Autodesk Inventor part; units mm, degrees
ref_plane "YZ Plane" through (0, 0, 0) normal (1, 0, 0) x (0, 1, 0)
ref_plane "XZ Plane" through (0, 0, 0) normal (0, 1, 0) x (-1, 0, 0)
ref_plane "XY Plane" through (0, 0, 0) normal (0, 0, 1) x (1, 0, 0)
sketch "Esquisse1" plane through (0, 0, 0) normal (0, 1, 0) x (-1, 0, 0)
  line L0 (21, 10.5) -> (-21, 10.5)
  line L1 (-21, 10.5) -> (-21, -10.5)
  line L2 (-21, -10.5) -> (21, -10.5)
  line L3 (21, -10.5) -> (21, 10.5)
  line L4 (29, 12.5) -> (-37, 12.5)
  line L5 (-37, 12.5) -> (-37, -12.5)
  line L6 (-37, -12.5) -> (29, -12.5)
  line L7 (29, -12.5) -> (29, 12.5)
  line L8 (-37, -12.5) -> (-46.0993, 12.5)
  line L9 (-46.0993, 12.5) -> (-37, 12.5)
  point P0 (0, 0)
  dimension "d0" = 20
  dimension "d1" = 42
  dimension "d2" = 21
  dimension "d3" = 10.5
  dimension "d4" = 21
  dimension "d5" = 8
  dimension "d6" = 2
  dimension "d7" = 2
  dimension "d8" = 16
extrude "Extrusion1" add sketch "Esquisse1" along normal mid plane 25
sketch "Esquisse2" plane through (37, -12.5, -12.5) normal (0.9397, 0, -0.342) x (-0.342, 0, -0.9397)
  line L0 (-26.6044, 25) -> (0, 0)
  line L1 (0, 0) -> (0, 25)
  line L2 (0, 25) -> (-26.6044, 0)
  arc A0 (-8.3022, 22.298) -> (-18.3022, 22.298) centre (-13.3022, 12.5) ccw
  line L3 (-18.3022, 22.298) -> (-8.3022, 22.298)
  line L4 (-8.3022, 22.298) -> (-8.3022, 2.702)
  line L5 (-8.3022, 2.702) -> (-18.3022, 2.702)
  line L6 (-18.3022, 2.702) -> (-18.3022, 22.298)
  arc A1 (-8.3022, 2.702) -> (-8.3022, 22.298) centre (-13.3022, 12.5) ccw
  arc A2 (-18.3022, 2.702) -> (-8.3022, 2.702) centre (-13.3022, 12.5) ccw
  arc A3 (-18.3022, 22.298) -> (-18.3022, 2.702) centre (-13.3022, 12.5) ccw
  point P0 (0.9086, 12.5)
  point P1 (-26.6044, 25)
  point P2 (-26.6044, 0)
  dimension "d11" = 22
  dimension "d13" = 10
extrude "Extrusion2" add sketch "Esquisse2" along normal blind 5 contours A3 L6 L0 | L0 L6 L2 A3 | L6 L3 L4 L2 L0 | L0 L2 L6 | L2 L6 A3 | L2 L4 L0 | L0 L4 L5 L6 L2 | A1 L2 L4 | L4 L2 A1 L0 | L0 A1 L4
sketch "Esquisse3" plane through (39.8395, -9.798, -4.6985) normal (0, -1, 0) x (0.9397, 0, -0.342)
  line L0 (5, 10) -> (0, 0)
  line L1 (0, 10) -> (5, 0)
  circle A0 centre (2.5, 5) radius 1.75
  point P0 (-39.0439, -9.2108)
  dimension "d16" = 3.5
extrude "Extrusion3" cut sketch "Esquisse3" against normal through all
sketch "Esquisse4" plane through (21, -12.5, 10.5) normal (-1, 0, 0) x (0, 0, 1)
  line L0 (-21, 3) -> (0, 3)
  line L1 (0, 3) -> (0, 6)
  line L2 (0, 6) -> (-21, 6)
  line L3 (-21, 6) -> (-21, 3)
  line L4 (-21, 0) -> (-21, 25)
  line L5 (0, 0) -> (0, 25)
  line L6 (0, 0) -> (-21, 0)
  point P0 (-10.5, 12.5)
  dimension "d19" = 3
  dimension "d20" = 3
extrude "Extrusion4" cut sketch "Esquisse4" against normal blind 7 contours L3 L2 L1 L0
sketch "Esquisse5" plane through (-21, -12.5, -10.5) normal (1, 0, 0) x (0, 0, -1)
  line L0 (-21, 6) -> (0, 6)
  line L1 (0, 6) -> (0, 3)
  line L2 (0, 3) -> (-21, 3)
  line L3 (-21, 3) -> (-21, 6)
  line L4 (-21, 25) -> (-21, 0)
  line L5 (0, 0) -> (0, 25)
  line L6 (0, 0) -> (-21, 0)
  point P0 (-10.5, 12.5)
  dimension "d23" = 3
  dimension "d24" = 3
extrude "Extrusion5" cut sketch "Esquisse5" against normal blind 7 contours L0 L1 L2 L3
sketch "Esquisse6" plane through (21, 12.5, -10.5) normal (-1, 0, 0) x (0, 0, 1)
  line L0 (21, -25) -> (0, 0)
  line L1 (0, -25) -> (21, 0)
  circle A0 centre (10.5, -12.5) radius 3
  dimension "d27" = 6
extrude "Extrusion6" cut sketch "Esquisse6" against normal through all
sketch "Esquisse7" plane through (21, 12.5, -10.5) normal (-1, 0, 0) x (0, 0, 1)
  circle A0 centre (10.5, -12.5) radius 3
  circle A1 centre (10.5, -12.5) radius 1.75
  circle A2 centre (10.5, -12.5) radius 3
  dimension "d30" = 0
  dimension "d31" = 3.5
extrude "Extrusion7" add sketch "Esquisse7" against normal blind 18
sketch "Esquisse8" plane through (21, 12.5, -10.5) normal (-1, 0, 0) x (0, 0, 1)
  circle A0 centre (10.5, -12.5) radius 3
  dimension "d34" = 6
extrude "Extrusion8" cut sketch "Esquisse8" against normal blind 3
sketch "Esquisse10" plane through (0, -12.5, 0) normal (0, -1, 0) x (1, 0, 0)
  line L0 (-21, -10.5) -> (-28, -10.5)
  line L1 (-28, -10.5) -> (-28, 10.5)
  line L2 (-28, 10.5) -> (-21, 10.5)
  line L3 (-21, 10.5) -> (-21, -10.5)
  line L4 (21, -10.5) -> (28, -10.5)
  line L5 (28, -10.5) -> (28, 10.5)
  line L6 (28, 10.5) -> (21, 10.5)
  line L7 (21, 10.5) -> (21, -10.5)
  line L8 (-28, -10.5) -> (-28, 10.5)
  line L9 (28, 10.5) -> (28, -10.5)
  line L10 (-28, -10.5) -> (-21, 0)
  line L11 (-21, 0) -> (-28, 10.5)
  line L12 (-28, 0) -> (-21, 10.5)
  line L13 (-21, -10.5) -> (-28, 0)
  line L14 (21, -10.5) -> (28, 0)
  line L15 (21, 0) -> (28, -10.5)
  line L16 (28, 10.5) -> (21, 0)
  line L17 (21, 10.5) -> (28, 0)
  circle A0 centre (-24.5, -5.25) radius 2
  circle A1 centre (24.5, -5.25) radius 2
  circle A2 centre (24.5, 5.25) radius 2
  circle A3 centre (-24.5, 5.25) radius 2
  point P0 (0, 0)
  dimension "d37" = 4
  dimension "d38" = 4
  dimension "d39" = 4
  dimension "d40" = 4
extrude "Extrusion9" cut sketch "Esquisse10" against normal through all contours A0 L10 L13 | L13 L10 A0 | A0 L13 L10 | L10 L13 A0 | A3 L12 L11 | L11 L12 A3 | A3 L11 L12 | L12 L11 A3 | A1 L15 L14 | L14 L15 A1 | L15 L14 A1 | A1 L14 L15 | A2 L17 L16 | L16 L17 A2 | L17 L16 A2 | A2 L16 L17
sketch "Esquisse11" plane through (37, 12.5, -12.5) normal (0, 0, -1) x (-1, 0, 0)
  line L0 (66, 0) -> (46, 0)
  line L1 (46, 0) -> (46, -13)
  line L2 (46, -13) -> (66, -13)
  line L3 (66, -13) -> (66, 0)
  line L4 (66, -25) -> (0, -25)
  line L5 (46, -13) -> (33, 0)
  line L6 (0, 0) -> (66, 0)
  line L7 (45, 0) -> (33, 0)
  point P0 (37, -12.5)
  dimension "d43" = 20
  dimension "d44" = 12
  dimension "d45" = 45
extrude "Extrusion10" cut sketch "Esquisse11" against normal through all
sketch "Esquisse12" plane through (-29, -12.5, 12.5) normal (0, 0, 1) x (1, 0, 0)
  line L0 (33, 25) -> (75.0993, 25)
  line L1 (75.0993, 0) -> (61.5, 0)
  line L2 (61.5, 0) -> (61.5, 25)
  line L3 (61.5, 25) -> (75.0993, 25)
  line L4 (75.0993, 25) -> (75.0993, 0)
  line L5 (57, 6) -> (57, 3)
  line L6 (66, 25) -> (66, 0)
  line L7 (61.5, 25) -> (0, 25)
  line L8 (0, 25) -> (0, 0)
  line L9 (0, 0) -> (61.5, 0)
  line L10 (61.5, 0) -> (61.5, 25)
  line L11 (75.0993, 0) -> (79.0103, 0)
  line L12 (79.0103, 0) -> (79.0103, 25)
  line L13 (79.0103, 25) -> (75.0993, 25)
  line L14 (75.0993, 25) -> (75.0993, 0)
  ellipse E0 centre (75.2481, 12.5) end of major axis (75.2481, 1.5) minor radius 3.7622 (76.9582, 2.702) -> (76.9582, 22.298) ccw
  point P0 (29, 12.5)
  dimension "d48" = 9
  dimension "d49" = 4.5
extrude "Extrusion12" cut sketch "Esquisse12" against normal through all contours L0 L6 L1 L2 | L0 L4 L1 L6 | L13 L12 L11 L4
sketch "Esquisse13" plane through (-29, -0.5, 12.5) normal (0, 0, 1) x (1, 0, 0)
  line L0 (0, -12) -> (0, 0)
  line L1 (61.5, -12) -> (0, -12)
  line L2 (0, -12) -> (0, -6)
  line L3 (0, -6) -> (61.5, -6)
  line L4 (61.5, -6) -> (61.5, -12)
  line L5 (61.5, 13) -> (0, 13)
  line L6 (0, 13) -> (0, -6)
  line L7 (0, -6) -> (61.5, -6)
  line L8 (61.5, -6) -> (61.5, 13)
  point P0 (29, 0.5)
  dimension "d54" = 6
extrude "Extrusion13" cut sketch "Esquisse13" against normal through all contours L0 L6 L5 L8 L3
sketch "Esquisse14" plane through (0, -12.5, 0) normal (0, -1, 0) x (1, 0, 0)
  circle A0 centre (-24.5, 5.25) radius 4
  circle A1 centre (-24.5, -5.25) radius 4
  circle A2 centre (24.5, 5.25) radius 4
  circle A3 centre (24.5, -5.25) radius 4
  circle A4 centre (-24.5, 5.25) radius 2
  circle A5 centre (-24.5, -5.25) radius 2
  circle A6 centre (24.5, 5.25) radius 2
  circle A7 centre (24.5, -5.25) radius 2
  point P0 (0, 0)
  dimension "d57" = 8
  dimension "d58" = 8
  dimension "d59" = 8
  dimension "d60" = 8
extrude "Extrusion14" cut sketch "Esquisse14" against normal blind 2
equation "\"d38\" = d37"
equation "\"d39\" = d37"
equation "\"d40\" = d37"
equation "\"d49\" = 0.5 * d48"
equation "\"d58\" = d57"
equation "\"d59\" = d57"
equation "\"d60\" = d57"
properties part number "forearm"
Source: CAD feature listing. Evaluate the final solid. Frame: model axes, mm. A direction names the side the tool comes from. Round coordinates to 2 decimals unless told otherwise and drop trailing zeros. Loops run counter-clockwise (first coordinate to the right, second up) from the corner with the lowest first, then second, coordinate; pieces in that order, holes last. Notation, with made-up numbers: M 86.25,-3 L 119.25,-3 A16 cw 119.25,1 Z; hole C 1.25,78 d7. An arc over 180 degrees is marked long. Use a Markdown table: item, result. Add a question column.
1. Cut plane C-C, the plane x = 24.5. Output: boundary loops of the cut face in (y, z).
2. Pull-direction query (Z, two-part tool) for faces 5 (the flat face through (8, -6.5, -11)), 6 (the cylindrical face through (-28.497, -11.514, -5.102)), 7 (the cylindrical face through (-26.087, -10.007, -6.467)); classes: +Z half, -Z half, draft (parallel to the pull), parting line (faces both ways), or undercut.
3. Cut plane B-B, the plane x = 12. Output: boundary loops of the cut face in (y, z), and give its area (3 significant figures).
4. Set-up query: faces 1 (the flat face through (24, -9.5, 0)), 2 (the flat face through (-26.5, -10.5, 6.2)), 3 (the flat face through (-21, -11, 0)), 4 (the flat face through (32.5, -10, 0)). Return all of +Z, -Z, +X, -X, +Y, -Y with unobstructed straight access to the full face (end or side cutting, diameter ignored); none if empty.
5. Contact query for flat-ended pins moving along their axis: pin 1 (9 mm diameter, centred on x = 24.5, z = -5.25, fed in from +Y); pin 2 (7 mm diameter, centred on x = -24.5, z = -5.25, fed in from -Y); pin 3 (2.5 mm diameter, centred on x = -24.5, z = 5.25, fed in from +Y); pin 4 (2 mm diameter, centred on x = -25.5, z = -0.5, fed in from +Y). Output: stop coordinate, or through.
6. Cut plane D-D, the plane y = -7.05. Output: boundary loops of the cut face in (x, z), and give its area (4 significant figures).
7. Cut plane A-A, the plane z = -5.25. Output: boundary loops of the cut face in (x, y).
8. Ray query, line 1 along Z through (x, y) = (-24.5, -11.7); line 2 along Z through (x, y) = (18.5, -7.9); line 3 along X through (y, z) = (-8.9, -0.5). Return the intervals inside material, ascending. Write a range as [from, to].
Solution:
| question | item | result |
|---|---|---|
| 1 | outline | M -12.5,-12.5 L -6.5,-12.5 L -6.5,-10.5 L -9.5,-10.5 L -9.5,-7.25 L -10.5,-7.25 L -10.5,-9.25 L -12.5,-9.25 Z; M -12.5,-1.25 L -10.5,-1.25 L -10.5,-3.25 L -9.5,-3.25 L -9.5,3.25 L -10.5,3.25 L -10.5,1.25 L -12.5,1.25 Z; M -12.5,9.25 L -10.5,9.25 L -10.5,7.25 L -9.5,7.25 L -9.5,10.5 L -6.5,10.5 L -6.5,12.5 L -12.5,12.5 Z |
| 2 | face 5 | draft |
| 2 | face 6 | undercut |
| 2 | face 7 | undercut |
| 3 | outline | M -12.5,-12.5 L -6.5,-12.5 L -6.5,-10.5 L -12.5,-10.5 Z; M -12.5,10.5 L -6.5,10.5 L -6.5,12.5 L -12.5,12.5 Z |
| 3 | area | 24.0 mm2 |
| 4 | face 1 | +Y |
| 4 | face 2 | -Y |
| 4 | face 3 | +Y, -Y |
| 4 | face 4 | +Z, -Z, +X, +Y, -Y |
| 5 | pin 1 | stops at y = -6.5 |
| 5 | pin 2 | stops at y = -10.5 |
| 5 | pin 3 | passes through |
| 5 | pin 4 | stops at y = -9.5 |
| 6 | outline | M -29,-12.5 L 32.5,-12.5 L 32.5,12.5 L -29,12.5 Z; hole M -28,-10.5 L 28,-10.5 L 28,10.5 L -28,10.5 Z |
| 6 | area | 361.5 mm2 |
| 7 | outline | M -29,-12.5 L -28.5,-12.5 L -28.5,-10.5 L -26.5,-10.5 L -26.5,-9.5 L -28,-9.5 L -28,-6.5 L -29,-6.5 Z; M -22.5,-10.5 L -21,-10.5 L -21,-9.5 L -22.5,-9.5 Z; M 21,-10.5 L 22.5,-10.5 L 22.5,-9.5 L 21,-9.5 Z; M 26.5,-10.5 L 28.5,-10.5 L 28.5,-12.5 L 32.5,-12.5 L 32.5,-6.5 L 28,-6.5 L 28,-9.5 L 26.5,-9.5 Z |
| 8 | line 1 | z = [-12.5, -9.25], [-1.25, 1.25], [9.25, 12.5] |
| 8 | line 2 | z = [-12.5, -10.5], [10.5, 12.5] |
| 8 | line 3 | x = [-29, -28], [28, 32.5] |
